Check sheet for the modelled part. Datum: model origin and axes. Units: mm. Face numbers are marked on the shaded views. A direction names the side the tool comes from. Coordinates: 2 decimals unless noted, no trailing zeros. Loops run counter-clockwise (first coordinate to the right, second up) from the corner with the lowest first, then second, coordinate; pieces in that order, holes last. Notation, with made-up numbers: (3, 44.25) - (14, 44.25) arc R18 ccw to (14, 51.25) - close; hole circle Ø7 at (28.25, 5.5). An arc over 180 degrees is marked (long way). Use a Markdown table: item, result. Add a question column.
1) Go/stop test with flat-tipped pins: P1, Ø12, axis at x = -30.5, z = 43, coming from the +Y side; P2, Ø1, axis at y = 23, z = 46.5, coming from the +X side; P3, Ø20.5, axis at x = 38.1, y = 25.4, coming from the +Z side; P4, Ø5, axis at y = -4.5, z = 49.5, coming from the +X side. Record where each tip stops, or that it passes through.
2) Thickness scan on line 1 (Y direction, x = 38, z = 18); line 2 (X direction, y = -25, z = 19); line 3 (Z direction, x = 40, y = 19). Record the ranges inside material, lowest first.
3) Sectioned sample at B-B, the plane y = 0. Enter the section's corners in (x, z), then the cut area to 3 significant figures.
4) Draft check along Y on the marked faces 3, 4, 5 and 6. Enter one of: pulls with the +Y half, pulls with the -Y half, needs draft (parallel to the pull), parting line crosses it, or undercut.
5) Tool access check on the marked faces 1 and 2. Record the directions out of +Z, -Z, +X, -X, +Y, -Y that give a thin tool (end or side, any length) a straight path to the whole face; none if there is none.
6) Sectioned sample at C-C, the plane z = 57. Enter the section's corners in (x, y), then the cut area to 3 significant figures.
7) Sectioned sample at A-A, the plane x = 38.1. Enter the section's corners in (y, z).
8) Sectioned sample at D-D, the plane x = -33.5. Enter the section's corners in (y, z), then the cut area to 3 significant figures.
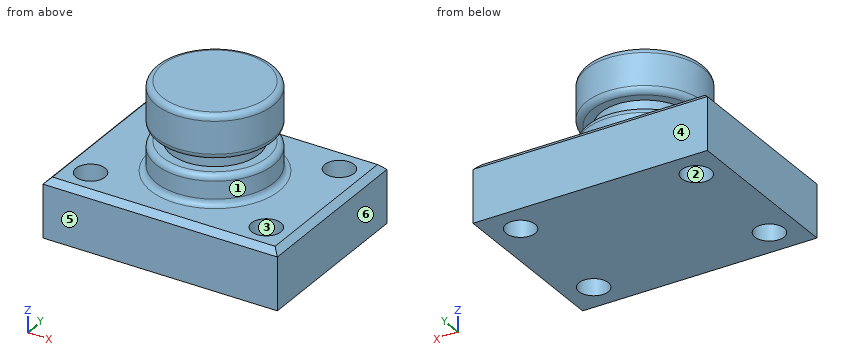
from build123d import *

# Parameters (mm, degrees)
F0_W     = 101.6
F0_H     = 76.2
F1_DEPTH = 25.4
F2_R     = 6.35
F3_DEPTH = 25.4
F4_W     = 25.4
F4_H     = 38.1
F6_W     = 25.4
F6_H     = 6.35
F8_SIZE  = 2.54
F9_R     = 2.54


with BuildPart() as f1:
    # F0 (on Top) → F1 (new body)
    with BuildSketch(Plane.XY):
        Rectangle(F0_W, F0_H)
    extrude(amount=F1_DEPTH)

    # F2 (on face) → F3 (cut)
    with BuildSketch(Plane.XY.offset(25.4)):
        with Locations((-38.1, 25.4)):
            Circle(F2_R)
        with Locations((38.1, 25.4)):
            Circle(F2_R)
        with Locations((38.1, -25.4)):
            Circle(F2_R)
        with Locations((-38.1, -25.4)):
            Circle(F2_R)
    extrude(amount=-F3_DEPTH, mode=Mode.SUBTRACT)

    # F4 (on Front) → F5 (revolve)
    with BuildSketch(Plane.XZ):
        with Locations((-12.7, 44.45)):
            Rectangle(F4_W, F4_H)
    revolve(axis=Axis((0, 0, 44.45), (0, 0, -1)))

    # F6 (on Right) → F7 (revolve, cut)
    with BuildSketch(Plane.YZ):
        with Locations((-31.75, 41.275)):
            Rectangle(F6_W, F6_H)
    revolve(axis=Axis((0, 0, 63.5), (0, 0, -1)), mode=Mode.SUBTRACT)

    # F8
    f8_edges = [f1.edges().sort_by_distance(p)[0] for p in [
        (0, 38.1, 25.4),
        (-50.8, 0, 25.4),
        (0, -38.1, 25.4),
        (50.8, 0, 25.4),
    ]]
    chamfer(f8_edges, length=F8_SIZE)

    # F9
    f9_edges = [f1.edges().sort_by_distance(p)[0] for p in [
        (25.4, 0, 25.4),
        (25.4, 0, 38.1),
        (25.4, 0, 44.45),
        (25.4, 0, 63.5),
    ]]
    fillet(f9_edges, radius=F9_R)


solid = f1.part
Solved:
| question | item | result |
|---|---|---|
| 1 | P1 | passes through |
| 1 | P2 | stops at x = 11.7 |
| 1 | P3 | stops at z = 25.4 |
| 1 | P4 | stops at x = 25.32 |
| 2 | line 1 | y = -38.1 to -31.75, -19.05 to 19.05, 31.75 to 38.1 |
| 2 | line 2 | x = -50.8 to -44.44, -31.76 to 31.76, 44.44 to 50.8 |
| 2 | line 3 | z = 0 to 25.4 |
| 3 | outline | (-50.8, 0) - (50.8, 0) - (50.8, 22.86) - (48.26, 25.4) - (27.94, 25.4) arc R2.54 cw to (25.4, 27.94) - (25.4, 35.56) arc R2.54 ccw to (22.86, 38.1) - (19.05, 38.1) - (19.05, 44.45) - (22.86, 44.45) arc R2.54 ccw to (25.4, 46.99) - (25.4, 60.96) arc R2.54 ccw to (22.86, 63.5) - (-22.86, 63.5) arc R2.54 ccw to (-25.4, 60.96) - (-25.4, 46.99) arc R2.54 ccw to (-22.86, 44.45) - (-19.05, 44.45) - (-19.05, 38.1) - (-22.86, 38.1) arc R2.54 ccw to (-25.4, 35.56) - (-25.4, 27.94) arc R2.54 cw to (-27.94, 25.4) - (-48.26, 25.4) - (-50.8, 22.86) - close |
| 3 | area | 4,420 mm2 |
| 4 | face 3 | undercut |
| 4 | face 4 | pulls with the +Y half |
| 4 | face 5 | pulls with the -Y half |
| 4 | face 6 | needs draft |
| 5 | face 1 | +Z |
| 5 | face 2 | +Z, -Z |
| 6 | outline | circle Ø50.8 at (0, 0) |
| 6 | area | 2,030 mm2 |
| 7 | outline | (-38.1, 0) - (-31.75, 0) - (-31.75, 25.4) - (-35.56, 25.4) - (-38.1, 22.86) - close; (-19.05, 0) - (19.05, 0) - (19.05, 25.4) - (-19.05, 25.4) - close; (31.75, 0) - (38.1, 0) - (38.1, 22.86) - (35.56, 25.4) - (31.75, 25.4) - close |
| 8 | outline | (-38.1, 0) - (-29.78, 0) - (-29.78, 25.4) - (-35.56, 25.4) - (-38.1, 22.86) - close; (-21.02, 0) - (21.02, 0) - (21.02, 25.4) - (-21.02, 25.4) - close; (29.78, 0) - (38.1, 0) - (38.1, 22.86) - (35.56, 25.4) - (29.78, 25.4) - close |
| 8 | area | 1,480 mm2 |
